Autodesk Fusion 360 part; units mm, degrees
sketch "Sketch1" plane through (0, 0, 0) normal (0, 0, 1) x (1, 0, 0)
  circle A0 centre (0, 0) radius 6
  circle A1 centre (0, 0) radius 2.85
  dimension "d1" = 12
  dimension "d2" = 5.7
extrude "Extrude1" add sketch "Sketch1" along normal blind 1.5 draft 2
sketch "Sketch2" plane through (0, 0, 0) normal (0, 0, -1) x (-1, 0, 0)
  circle A0 centre (0, 0) radius 2.85
  circle A1 centre (0, 0) radius 6
  circle A2 centre (0, 0) radius 3.5
  dimension "d5" = 7
extrude "Extrude2" add sketch "Sketch2" along normal blind 6.5 contours A2
sketch "Sketch3" plane through (0, 0, -6.5) normal (0, 0, -1) x (-1, 0, 0)
  circle A0 centre (0, 0) radius 2.85
  circle A1 centre (0, 0) radius 3.5
  circle A2 centre (0, 0) radius 3.5
  circle A3 centre (0, 0) radius 1.5
  dimension "d8" = 3
extrude "Extrude3" add sketch "Sketch3" against normal blind 2 contours A0
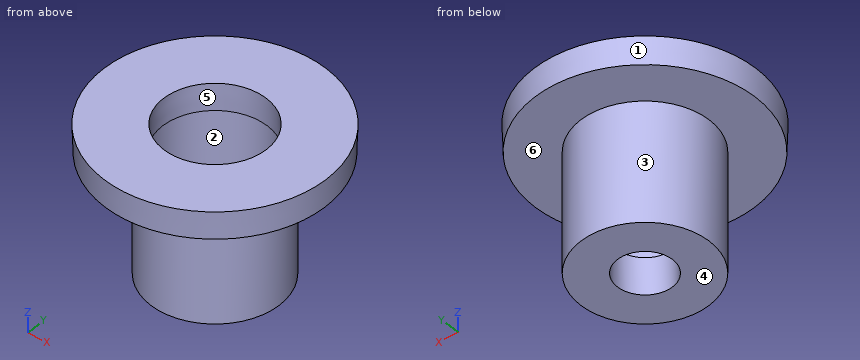
The listing builds one solid part. Answer for the finished solid, in the listing's coordinates (mm). Face numbers are marked on the shaded views. A direction names the side the tool comes from. Give positions to 0.01 mm unless a question says otherwise; leave off trailing zeros. Write each loop counter-clockwise with the first axis right and the second up, starting at its lowest first coordinate (ties: lowest second). Pieces come first, ordered by that corner, then holes.
Item 1: Determine the mould class of the marked faces 1, 2 and 3 for opening direction Z: released by +Z, released by -Z, zero draft, split by the parting line, or undercut.
Item 2: Flat-ended cylindrical pins translate along their axes: P1, Ø1.8, axis at x = 0, y = 0, coming from the -Z side; P2, Ø4, axis at x = -0.5, z = -2.5, coming from the +Y side; P3, Ø3, axis at x = -2, z = -2.5, coming from the -Y side; P4, Ø3, axis at x = 0, y = 0.5, coming from the +Z side. Find the tip coordinate at first contact, or state that the pin passes through.
Item 3: Which of the six approach directions +Z, -Z, +X, -X, +Y, -Y give full straight-line access (tool end or side, diameter ignored) to the marked faces 4, 5 and 6?
Item 4: Section C-C, the plane z = -5 is taken. Write down the section's boundary in (x, y), plus the area to 3 significant figures.
Item 5: Find the intervals of material crossed by line 1 along Y through (x, z) = (0, -5.4); line 2 along Z through (x, y) = (3.75, -2.5); line 3 along Z through (x, y) = (-2.25, -1.25), in increasing order.
Item 6: Section D-D, the plane z = -4 is taken. Write down the section's boundary in (x, y), plus the area to 3 significant figures.
Item 7: Section A-A, the plane x = 0 is taken. Write down the section's boundary in (y, z).
Completed:
1. face 1: released by -Z
1. face 2: undercut
1. face 3: zero draft
2. P1: passes through
2. P2: stops at y = 3.5
2. P3: stops at y = -3.46
2. P4: stops at z = -4.5
3. face 4: -Z, +X, -X, +Y, -Y
3. face 5: none
3. face 6: -Z
4. outline: circle Ø7 at (0, 0); hole circle Ø3 at (0, 0)
4. area: 31.4 mm2
5. line 1: y = -3.5 to -1.5, 1.5 to 3.5
5. line 2: z = 0 to 1.5
5. line 3: z = -6.5 to -4.5
6. outline: circle Ø7 at (0, 0); hole circle Ø5.7 at (0, 0)
6. area: 13.0 mm2
7. outline: (-6.05, 1.5) - (-6, 0) - (-3.5, 0) - (-3.5, -6.5) - (-1.5, -6.5) - (-1.5, -4.5) - (-2.85, -4.5) - (-2.85, 0) - (-2.8, 1.5) - close; (1.5, -6.5) - (3.5, -6.5) - (3.5, 0) - (6, 0) - (6.05, 1.5) - (2.8, 1.5) - (2.85, 0) - (2.85, -4.5) - (1.5, -4.5) - close
